Geometry check sheet. Reference: drawing and pictorial views, mm from the part's lowest x, y, z. A direction names the side the tool comes from. Give positions to 0.01 mm unless a question says otherwise; leave off trailing zeros. Order: outer loops, then holes, each group sorted by start corner. A loop starts at its lowest first (then second) coordinate and runs counter-clockwise, first axis right, second up. Notation, with made-up numbers: (59.25, -38) - (115.25, -38) arc R13 cw to (115.25, -34) - close; hole circle Ø8 at (35.25, -21). An arc over 180 degrees is marked (long way). Answer as a JSON object with one key per item and string values.
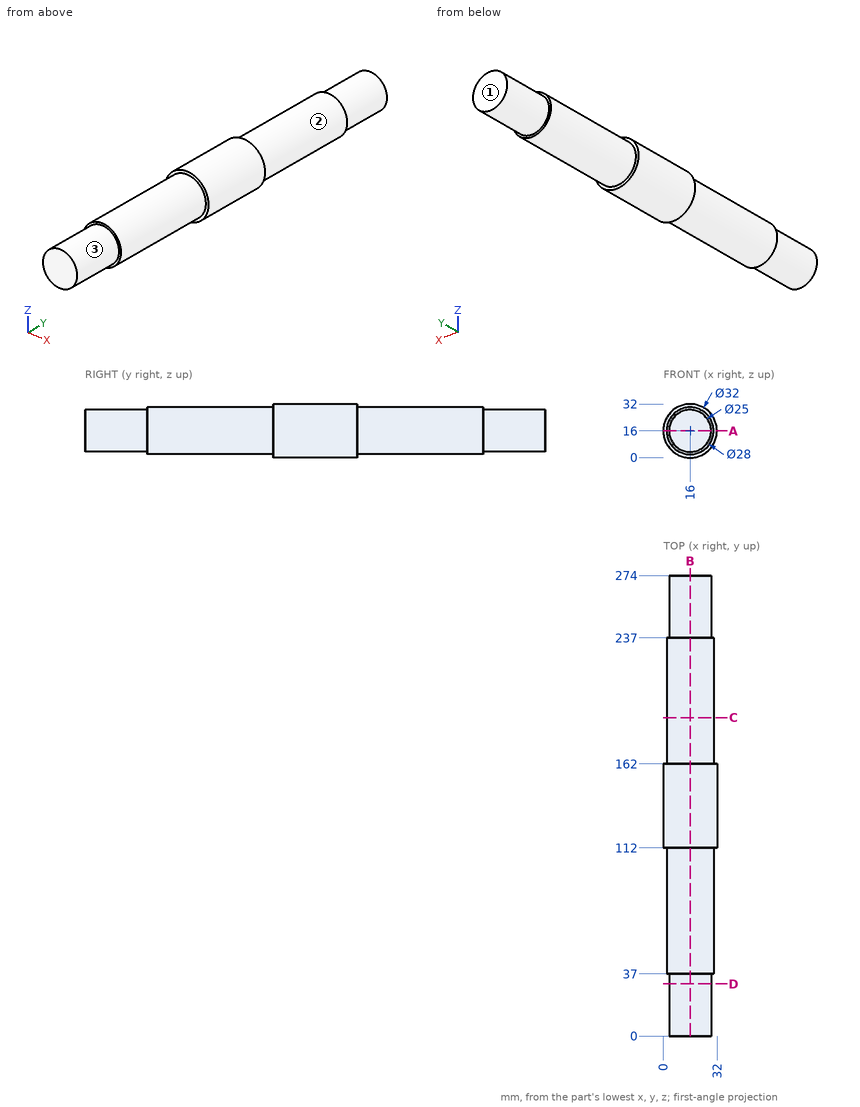
(1) Section check D-D (y = 31). Record the cut outline in (x, z).
Computed values:
{"outline": "circle Ø25 at (16, 16)"}
(2) Gauge pin test, flat ends, axial feed: pin 1 Ø10 at (y, z) = (151.5, 27) entering from -X; pin 2 Ø3 at (y, z) = (230.5, 19.5) entering from +X; pin 3 Ø12 at (x, y) = (11.5, 35) entering from -Z. Record the tip position at first contact, or that the pin passes through.
Computed values:
{"pin 1": "stops at x = 1.17", "pin 2": "stops at x = 29.86", "pin 3": "stops at z = 2"}
(3) Access from +Z, -Z, +X, -X, +Y, -Y to the whole of each face (thin tool, end or side, straight path). Record for the marked faces 1, 2 and 3.
Computed values:
{"face 1": "+Z, -Z, +X, -X, +Y", "face 2": "+Y", "face 3": "-Y"}
(4) Section check C-C (y = 189.5). Record the cut outline in (x, z), then the cut area to 3 significant figures.
Computed values:
{"outline": "circle Ø28 at (16, 16)", "area": "616 mm²"}
(5) Section check A-A (z = 16). Record the cut outline in (x, y), then the cut area to 3 significant figures.
Computed values:
{"outline": "(0, 112) - (2, 112) - (2, 37) - (3.5, 37) - (3.5, 0) - (28.5, 0) - (28.5, 37) - (30, 37) - (30, 112) - (32, 112) - (32, 162) - (30, 162) - (30, 237) - (28.5, 237) - (28.5, 274) - (3.5, 274) - (3.5, 237) - (2, 237) - (2, 162) - (0, 162) - close", "area": "7,650 mm²"}
(6) Material ranges on line 1 along Z through (x, y) = (16, 53); line 2 along Y through (x, z) = (6.5, 27.5); line 3 along Z through (x, y) = (15, 159.5), recorded low to high. Write a range as [from, to].
Computed values:
{"line 1": "z = [2, 30]", "line 2": "y = [112, 162]", "line 3": "z = [0.03, 31.97]"}
(7) Section check B-B (x = 16). Record the cut outline in (y, z), then the cut area to 3 significant figures.
Computed values:
{"outline": "(0, 3.5) - (37, 3.5) - (37, 2) - (112, 2) - (112, 0) - (162, 0) - (162, 2) - (237, 2) - (237, 3.5) - (274, 3.5) - (274, 28.5) - (237, 28.5) - (237, 30) - (162, 30) - (162, 32) - (112, 32) - (112, 30) - (37, 30) - (37, 28.5) - (0, 28.5) - close", "area": "7,650 mm²"}
